Input: dimensioned drawing with shaded views. Units: mm. Origin: part minimum x, y, z. Round coordinates to 2 decimals unless told otherwise and drop trailing zeros. Order: outer loops, then holes, each group sorted by start corner. A loop starts at its lowest first (then second) coordinate and runs counter-clockwise, first axis right, second up. Notation, with made-up numbers: M 27,52.25 L 41,52.25 A27 cw 41,70.25 Z; hole C -29,76.5 d10. An arc over 180 degrees is marked long. Answer as CSV lines item,"result". Start each with the question number.
Item 1: First-contact query: P1, Ø3, axis at x = 206, z = 2.5, coming from the -Y side; P2, Ø3, axis at y = 261, z = 3.5, coming from the +X side. Flat tips, straight axial feed; report the tip coordinate or a pass-through.
Item 2: Section query B-B on z = 4.5. State how many separate pieces and enclosed holes the cut face has, plus the area to 3 significant figures.
Item 3: Section query A-A on x = 158.75. Return the cut outline in (y, z).
Item 4: Line query: line 1 (Y direction, x = 315.5, z = 5.75); line 2 (X direction, y = 516.89, z = 3); line 3 (Y direction, x = 158.75, z = 4.5). Output: solid intervals per line, ascending. Write a range as [from, to].
Item 5: Section query D-D on y = 458. Return the cut outline in (x, z).
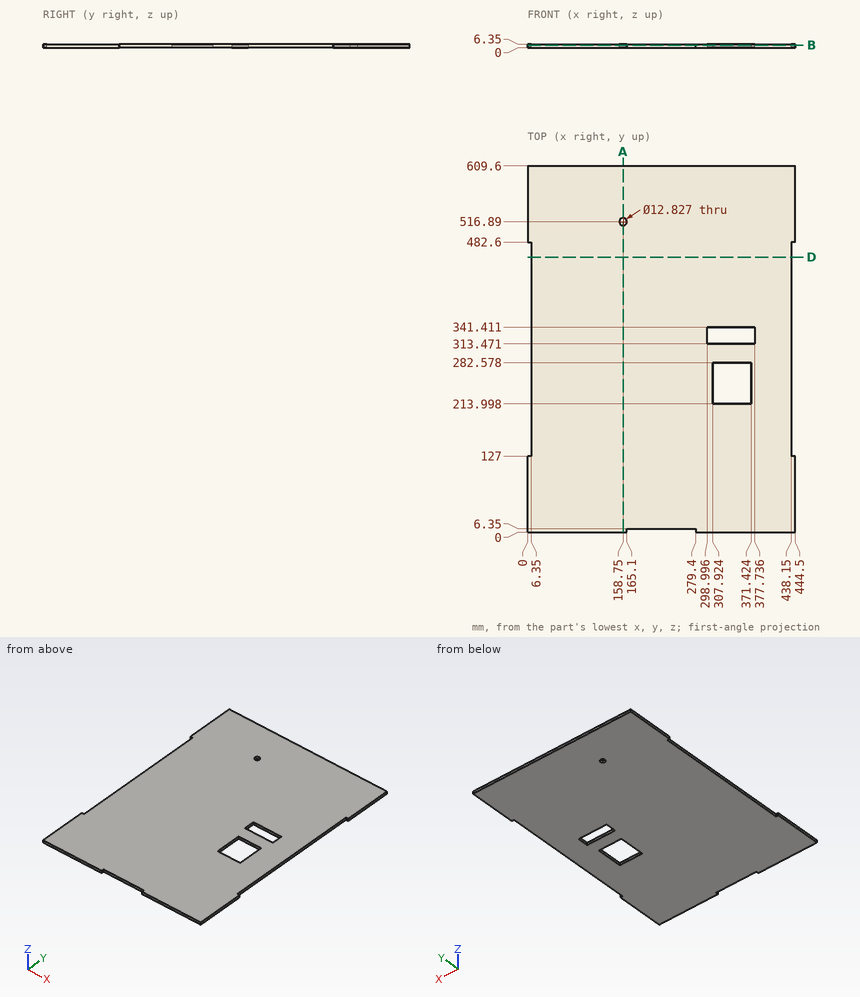
Results:
1,P1,"y = 6.35"
1,P2,"x = 438.15"
2,separate pieces,"1"
2,enclosed holes,"3"
2,area,"259,000 mm^2"
3,outline,"M 0,0 L 510.48,0 L 510.48,6.35 L 0,6.35 Z; M 523.3,0 L 609.6,0 L 609.6,6.35 L 523.3,6.35 Z"
4,line 1,"[0, 214], [282.58, 313.47], [341.41, 609.6]"
4,line 2,"[0, 152.34], [165.16, 444.5]"
4,line 3,"[0, 510.48], [523.3, 609.6]"
5,outline,"M 6.35,0 L 438.15,0 L 438.15,6.35 L 6.35,6.35 Z"
